Study the drawing (mm; zero at the part's minimum x, y, z) and answer. Round coordinates to 2 decimals unless told otherwise and drop trailing zeros. Write each loop counter-clockwise with the first axis right and the second up, starting at its lowest first coordinate (ties: lowest second). Pieces come first, ordered by that corner, then holes.
(1) A cutting plane is placed at C-C, the plane z = 45. Give the vertices of the cut face in (x, y).
(2) Find the intervals of material crossed by probe 1 along Z at (x, y) = (7.25, 0.95) (1 decimal); probe 2 along X at (y, z) = (1.6, 45); probe 3 along X at (y, z) = (2.25, 46) (1 decimal), in increasing order.
(3) A cutting plane is placed at B-B, the plane y = 0.9. Give the number of separate pieces and of enclosed holes in the cut face, and give its area (3 significant figures).
(4) This flat-tipped pin is pushed along its axis until it touches: pin 1 Ø1.5 at (y, z) = (1.5, 44) entering from +X. Where does it stop, or does it pass through?
(5) A cutting plane is placed at D-D, the plane x = 12.25. Give the vertices of the cut face in (y, z) (1 decimal), and give its area (3 significant figures).
(6) A cutting plane is placed at A-A, the plane z = 30. Give the vertices of the cut face in (x, y), and give its area (3 significant figures).
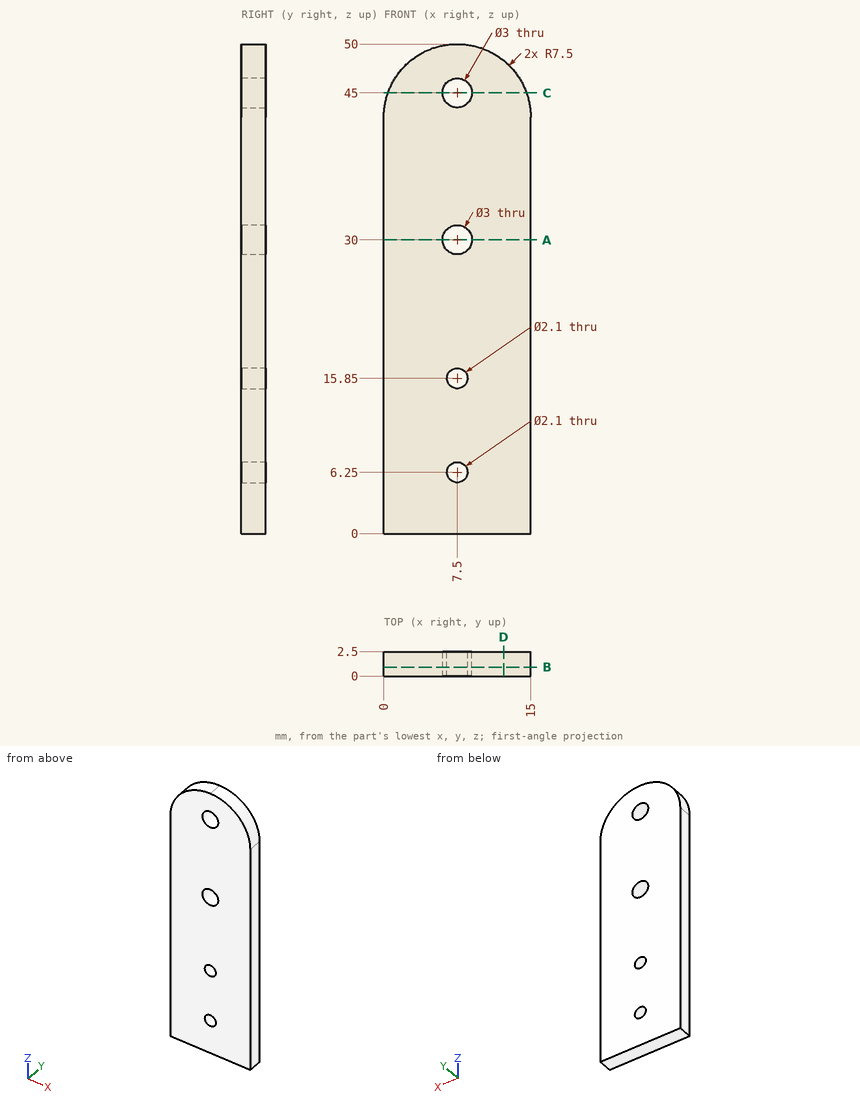
Solutions:
1. outline: (0.43, 0) - (6, 0) - (6, 2.5) - (0.43, 2.5) - close; (9, 0) - (14.57, 0) - (14.57, 2.5) - (9, 2.5) - close
2. probe 1: z = 0 to 5.2, 7.3 to 14.8, 16.9 to 28.5, 31.5 to 43.5, 46.5 to 50
2. probe 2: x = 0.43 to 6, 9 to 14.57
2. probe 3: x = 0.9 to 6.4, 8.6 to 14.1
3. separate pieces: 1
3. enclosed holes: 4
3. area: 705 mm2
4. pin 1: stops at x = 14.96
5. outline: (0, 0) - (2.5, 0) - (2.5, 48.3) - (0, 48.3) - close
5. area: 121 mm2
6. outline: (0, 0) - (6, 0) - (6, 2.5) - (0, 2.5) - close; (9, 0) - (15, 0) - (15, 2.5) - (9, 2.5) - close
6. area: 30.0 mm2
